Geometry check sheet. Reference: the model listing, model coordinates, mm. A direction names the side the tool comes from. Coordinates: 2 decimals unless noted, no trailing zeros. Write each loop counter-clockwise with the first axis right and the second up, starting at its lowest first coordinate (ties: lowest second). Pieces come first, ordered by that corner, then holes. Notation, with made-up numbers: M 37,88 L 92,88 A15 cw 92,103 Z; hole C 21.5,60 d11. An arc over 180 degrees is marked long. Put each result on its own line as item: value. Start each with the question number.
1) Scan lines: line 1 along Y through (x, z) = (17, -304) (1 decimal); line 2 along X through (y, z) = (128, -245.5); line 3 along Y through (x, z) = (0.8, -412.75). Record each from-to range of solid material in increasing order.
2) Cross-section at A-A on x = 21.5. Record the cut outline in (y, z) (1 decimal), plus the area to 3 significant figures.
3) Mould release check, pull along Y, two halves, no side actions. Record for faces 1 (the flat face through (1.588, 114, -407)), 2 (the cylindrical face through (0.8, 168.6, -617.2)), 3 (the flat face through (14, 235.077, -407)), 4 (the flat face through (0.4, 171.8, -825.5)): released by +Y, released by -Y, zero draft, split by the parting line, or undercut.
4) Set-up check for faces 5 (the flat face through (14, -1.588, -408)), 6 (the flat face through (0.411, 52.647, -24.797)): record each of +Z, -Z, +X, -X, +Y, -Y from which the full face is reachable in a straight line by a thin tool's end or side.
5) Gauge pin test, flat end, axial feed: pin 1 (1.5 mm diameter, centred on y = 36, z = -494, fed in from +X). Record the tip position at first contact, or that the pin passes through.
from build123d import *

# Parameters (mm, degrees)
BASE_FLANGE2_DEPTH                                 = 825.5
SKETCH1_R                                          = 3.175
SKETCH1_R_2                                        = 2.413
SKETCH1_R_3                                        = 5.55625
SKETCH1_R_4                                        = 2.5527
SKETCH1_R_5                                        = 2.0447
SKETCH1_R_6                                        = 14.28115
SKETCH1_R_7                                        = 11.10615
SKETCH1_R_8                                        = 1.5875
SKETCH1_R_9                                        = 9.525
SKETCH1_R_10                                       = 1.27
SKETCH1_R_11                                       = 14.2875
SKETCH1_R_12                                       = 4.7625
CUT_EXTRUDE3_DEPTH                                 = 859.694710551
CSK_FOR_10_FLAT_HEAD_MACHINE_SCREW_100_D           = 4.9784
CSK_FOR_10_FLAT_HEAD_MACHINE_SCREW_100_CSINK_D     = 9.779
CSK_FOR_10_FLAT_HEAD_MACHINE_SCREW_100_CSINK_ANGLE = 100
CSK_FOR_10_FLAT_HEAD_MACHINE_SCREW_2_AT_COUNT      = 2
CSK_FOR_10_FLAT_HEAD_MACHINE_SCREW_2_AT_PITCH      = 50.701163977
CSK_FOR_10_FLAT_HEAD_MACHINE_SCREW_3_COUNT         = 2
CSK_FOR_10_FLAT_HEAD_MACHINE_SCREW_3_PITCH         = 50.701163977
SKETCH10_R                                         = 0.635
CUT_EXTRUDE4_DEPTH                                 = 860.130662682
F_8_CLEARANCE_HOLE1_D                              = 4.9149
F_8_CLEARANCE_HOLE1_DEPTH                          = 1.5875
F_8_CLEARANCE_HOLE2_D                              = 4.9149
F_8_CLEARANCE_HOLE2_DEPTH                          = 1.5875


# Sheet-metal steps are written as plain solids
with BuildPart() as part:
    # Sketch3 → Base-Flange2 (new body)
    with BuildSketch(Plane.XY):
        with BuildLine():
            Line((3.175, 233.4895), (25.4, 233.4895))
            Line((25.4, 233.4895), (25.4, 235.077))
            Line((25.4, 235.077), (3.175, 235.077))
            ThreePointArc((3.175, 235.077), (0.92993597, 234.14706403), (0, 231.902))
            Line((0, 231.902), (0, 0))
            ThreePointArc((0, 0), (0.92993597, -2.24506403), (3.175, -3.175))
            Line((3.175, -3.175), (25.4, -3.175))
            Line((25.4, -3.175), (25.4, -1.5875))
            Line((25.4, -1.5875), (3.175, -1.5875))
            ThreePointArc((3.175, -1.5875), (2.052467985, -1.122532015), (1.5875, 0))
            Line((1.5875, 0), (1.5875, 231.902))
            ThreePointArc((1.5875, 231.902), (2.052467985, 233.024532015), (3.175, 233.4895))
        make_face()
    extrude(amount=-BASE_FLANGE2_DEPTH)

    # Sketch1 → Cut-Extrude3 (cut, through all)
    with BuildSketch(Plane(origin=(0, 0, 0), x_dir=(0, 0, -1), z_dir=(1, 0, 0))):
        with Locations(Location((516.509, 31.75, 0), (0, 0, 90))):
            Circle(SKETCH1_R)
        with Locations(Location((308.991, 31.75, 0), (0, 0, 90))):
            Circle(SKETCH1_R)
        with Locations(Location((103.492550911, 60.630923565, 0), (0, 0, 90))):
            Circle(SKETCH1_R)
        with Locations(Location((722.007449089, 60.630923565, 0), (0, 0, 90))):
            Circle(SKETCH1_R)
        with Locations(Location((412.75, 6.35, 0), (0, 0, 90))):
            Circle(SKETCH1_R_2)
        with Locations(Location((412.75, 88.9, 0), (0, 0, 90))):
            Circle(SKETCH1_R_2)
        with Locations(Location((622.478249316, 6.35, 0), (0, 0, 90))):
            Circle(SKETCH1_R_2)
        with Locations(Location((612.465522577, 88.9, 0), (0, 0, 90))):
            Circle(SKETCH1_R_2)
        with Locations(Location((203.021750684, 6.35, 0), (0, 0, 90))):
            Circle(SKETCH1_R_2)
        with Locations(Location((101.978503418, 46.225723918, 0), (0, 0, 90))):
            Circle(SKETCH1_R)
        with Locations(Location((723.521496582, 46.225723918, 0), (0, 0, 90))):
            Circle(SKETCH1_R)
        with Locations(Location((213.034477423, 88.9, 0), (0, 0, 90))):
            Circle(SKETCH1_R_2)
        with Locations(Location((359.180063087, 107.266959746, 0), (0, 0, 90))):
            Circle(SKETCH1_R_3)
        with Locations(Location((342.162063087, 114.251959746, 0), (0, 0, 90))):
            Circle(SKETCH1_R_4)
        with Locations(Location((342.162063087, 108.409959746, 0), (0, 0, 90))):
            Circle(SKETCH1_R_5)
        with Locations(Location((342.162063087, 177.751959746, 0), (0, 0, 90))):
            Circle(SKETCH1_R_4)
        with Locations(Location((342.162063087, 183.593959746, 0), (0, 0, 90))):
            Circle(SKETCH1_R_5)
        with Locations(Location((359.180063087, 184.736959746, 0), (0, 0, 90))):
            Circle(SKETCH1_R_3)
        with Locations(Location((384.580063087, 184.736959746, 0), (0, 0, 90))):
            Circle(SKETCH1_R_3)
        with Locations(Location((409.980063087, 184.736959746, 0), (0, 0, 90))):
            Circle(SKETCH1_R_3)
        with Locations(Location((431.062063087, 184.736959746, 0), (0, 0, 90))):
            Circle(SKETCH1_R_4)
        with Locations(Location((431.062063087, 190.578959746, 0), (0, 0, 90))):
            Circle(SKETCH1_R_5)
        with Locations(Location((431.062063087, 107.266959746, 0), (0, 0, 90))):
            Circle(SKETCH1_R_4)
        with Locations(Location((431.062063087, 101.424959746, 0), (0, 0, 90))):
            Circle(SKETCH1_R_5)
        with Locations(Location((412.75, 146.001959746, 0), (0, 0, 90))):
            Circle(SKETCH1_R_6)
        with Locations(Location((372.0338, 146.001959746, 0), (0, 0, 90))):
            Circle(SKETCH1_R_7)
        with Locations(Location((384.580063087, 107.266959746, 0), (0, 0, 90))):
            Circle(SKETCH1_R_3)
        with Locations(Location((409.980063087, 107.266959746, 0), (0, 0, 90))):
            Circle(SKETCH1_R_3)
        with Locations(Location((480.14255, 67.39255, 0), (0, 0, 90))):
            Circle(SKETCH1_R_8)
        with Locations(Location((510.45745, 67.39255, 0), (0, 0, 90))):
            Circle(SKETCH1_R_8)
        with Locations(Location((510.45745, 97.70745, 0), (0, 0, 90))):
            Circle(SKETCH1_R_8)
        with Locations(Location((480.14255, 97.70745, 0), (0, 0, 90))):
            Circle(SKETCH1_R_8)
        with Locations(Location((495.3, 82.55, 0), (0, 0, 90))):
            Circle(SKETCH1_R_9)
        with Locations(Location((636.250067105, 173.192896507, 0), (0, 0, 90))):
            Circle(SKETCH1_R_10)
        with Locations(Location((603.25, 171.694372229, 0), (0, 0, 90))):
            Circle(SKETCH1_R_11)
        with Locations(Location((570.249932895, 173.192896507, 0), (0, 0, 90))):
            Circle(SKETCH1_R_10)
        with Locations(Location((603.25, 211.684500783, 0), (0, 0, 90))):
            Circle(SKETCH1_R_10)
        with Locations(Location((544.318501255, 152.527, 0), (0, 0, 90))):
            Circle(SKETCH1_R_12)
        Polygon((825.5, -3.175), (775.673017562, -3.175), (825.5, 107.95), align=None)
        Polygon((0, 107.95), (49.826982438, -3.175), (0, -3.175), align=None)
    extrude(amount=CUT_EXTRUDE3_DEPTH, mode=Mode.SUBTRACT)

    # CSK for _10 Flat Head Machine Screw _100 (through all)
    with Locations(Plane.ZY):
        with Locations((-510.45745, 97.70745), (-480.14255, 97.70745), (-480.14255, 67.39255), (-510.45745, 67.39255)):
            CounterSinkHole(CSK_FOR_10_FLAT_HEAD_MACHINE_SCREW_100_D / 2, CSK_FOR_10_FLAT_HEAD_MACHINE_SCREW_100_CSINK_D / 2, counter_sink_angle=CSK_FOR_10_FLAT_HEAD_MACHINE_SCREW_100_CSINK_ANGLE)

    # Sketch8 → CSK for _10 Flat Head Machine Screw  2 (revolve, cut)
    with BuildSketch(Plane(origin=(1.5875, 211.684500783, -603.25), x_dir=(0, 0, -1), z_dir=(0, 1, 0))):
        Polygon((0, 0), (0, 1.5875), (2.4892, 1.5875), (2.4892, 2.014090845), (4.8895, 0), align=None)
    csk_for_10_flat_head_machine_screw_2 = revolve(axis=Axis((7.9375, 211.684500783, -603.25), (-1, 0, 0)), mode=Mode.SUBTRACT)

    # CSK for _10 Flat Head Machine Screw 2 at: CSK for _10 Flat Head Machine Screw  2 ×2
    with Locations(*[Vector(0, -0.7591858106628883, -0.6508739546856467) * (i * CSK_FOR_10_FLAT_HEAD_MACHINE_SCREW_2_AT_PITCH) for i in range(1, CSK_FOR_10_FLAT_HEAD_MACHINE_SCREW_2_AT_COUNT)]):
        add(csk_for_10_flat_head_machine_screw_2, mode=Mode.SUBTRACT)

    # CSK for _10 Flat Head Machine Screw  3: CSK for _10 Flat Head Machine Screw  2 ×2
    with Locations(*[Vector(0, -0.7591858106628849, 0.6508739546856506) * (i * CSK_FOR_10_FLAT_HEAD_MACHINE_SCREW_3_PITCH) for i in range(1, CSK_FOR_10_FLAT_HEAD_MACHINE_SCREW_3_COUNT)]):
        add(csk_for_10_flat_head_machine_screw_2, mode=Mode.SUBTRACT)

    # Sketch10 → Cut-Extrude4 (cut, through all)
    with BuildSketch(Plane(origin=(0, -1.5875, 0), x_dir=(1, 0, 0), z_dir=(0, 1, 0))):
        with Locations(Location((14.2875, 443.018983217, 0), (0, 0, 180))):
            Circle(SKETCH10_R)
        with Locations(Location((14.2875, 455.718983217, 0), (0, 0, 180))):
            Circle(SKETCH10_R)
        with Locations(Location((14.2875, 468.418983217, 0), (0, 0, 180))):
            Circle(SKETCH10_R)
        with Locations(Location((14.2875, 481.118983217, 0), (0, 0, 180))):
            Circle(SKETCH10_R)
        with Locations(Location((14.2875, 493.818983217, 0), (0, 0, 180))):
            Circle(SKETCH10_R)
        with Locations(Location((14.2875, 506.518983217, 0), (0, 0, 180))):
            Circle(SKETCH10_R)
        with Locations(Location((14.2875, 519.218983217, 0), (0, 0, 180))):
            Circle(SKETCH10_R)
        with Locations(Location((14.2875, 531.918983217, 0), (0, 0, 180))):
            Circle(SKETCH10_R)
    extrude(amount=-CUT_EXTRUDE4_DEPTH, mode=Mode.SUBTRACT)

    # #8 Clearance Hole1
    with Locations(Plane(origin=(0, -1.5875, 0), x_dir=(1, 0, 0), z_dir=(0, 1, 0))):
        with Locations((14.2875, 531.918983217), (14.2875, 519.218983217), (14.2875, 506.518983217), (14.2875, 493.818983217), (14.2875, 481.118983217), (14.2875, 468.418983217), (14.2875, 455.718983217), (14.2875, 443.018983217)):
            Hole(F_8_CLEARANCE_HOLE1_D / 2, depth=F_8_CLEARANCE_HOLE1_DEPTH)

    # #8 Clearance Hole2
    with Locations(Plane(origin=(0, 233.4895, 0), x_dir=(-1, 0, 0), z_dir=(0, -1, 0))):
        with Locations((-14.2875, 558.8), (-14.2875, 546.1), (-14.2875, 571.5), (-14.2875, 584.2), (-14.2875, 596.9), (-14.2875, 609.6), (-14.2875, 622.3), (-14.2875, 635)):
            Hole(F_8_CLEARANCE_HOLE2_D / 2, depth=F_8_CLEARANCE_HOLE2_DEPTH)


solid = part.part
Answer key:
1. line 1: y = -3.2 to -1.6, 233.5 to 235.1
1. line 2: x = 0 to 1.59
1. line 3: y = -2.11 to 3.94, 8.76 to 86.49, 91.31 to 102.45, 112.08 to 131.72, 160.28 to 179.92, 189.55 to 234.01
2. outline: M -3.2,-775.7 L -1.6,-776.4 L -1.6,-49.1 L -3.2,-49.8 Z; M 233.5,-825.5 L 235.1,-825.5 L 235.1,0 L 233.5,0 Z
2. area: 2,460 mm²
3. face 1: undercut
3. face 2: undercut
3. face 3: released by +Y
3. face 4: zero draft
4. face 5: +Z, -Z, +X
4. face 6: +Z, +X, -X, -Y
5. pin 1: stops at x = 1.59
